Input: part model. Units: mm. Frame: model coordinates. A direction names the side the tool comes from. Coordinates: 2 decimals unless noted, no trailing zeros. Write each loop counter-clockwise with the first axis right and the second up, starting at its lowest first coordinate (ties: lowest second). Pieces come first, ordered by that corner, then holes. Notation, with made-up numbers: (84, 26) - (133, 26) arc R31 ccw to (133, 64) - close; hole circle Ø2 at (74.5, -17.5). An arc over 180 degrees is marked (long way). Use CSV: the item, a comma, the result in double quotes.
```python
from build123d import *

# Parameters (mm, degrees)
CROQUIS1_R              = 2
SALIENTE_EXTRUIR1_DEPTH = 7
SALIENTE_EXTRUIR2_DEPTH = 5
SALIENTE_EXTRUIR3_DEPTH = 5
SALIENTE_EXTRUIR4_DEPTH = 5
CROQUIS6_R              = 2
CORTAR_EXTRUIR1_DEPTH   = 20
SALIENTE_EXTRUIR5_DEPTH = 5
CROQUIS8_R              = 2
CORTAR_EXTRUIR3_DEPTH   = 20
CORTAR_EXTRUIR4_DEPTH   = 20
CROQUIS10_R             = 2
CORTAR_EXTRUIR5_DEPTH   = 5
CROQUIS12_R             = 2
CORTAR_EXTRUIR6_DEPTH   = 5
CROQUIS13_R             = 2
CORTAR_EXTRUIR7_DEPTH   = 45


with BuildPart() as part:
    # Croquis1 → Saliente-Extruir1 (new body)
    with BuildSketch(Plane.XY):
        with BuildLine():
            Line((0, 161.361306161), (59.639031754, 161.361306161))
            ThreePointArc((59.639031754, 161.361306161), (66.710099565, 158.432373972), (69.639031754, 151.361306161))
            Line((69.639031754, 151.361306161), (69.639031754, 150.370999495))
            ThreePointArc((69.639031754, 150.370999495), (70.657777859, 141.400946832), (73.662123993, 132.887804479))
            ThreePointArc((73.662123993, 132.887804479), (90.138531177, 101.602103147), (108.605347016, 71.44843315))
            ThreePointArc((108.605347016, 71.44843315), (129.868212527, 5.85212568), (114.591350051, -61.390736219))
            ThreePointArc((114.591350051, -61.390736219), (94.163470567, -82.020942746), (65.787006352, -88.15934321))
            ThreePointArc((65.787006352, -88.15934321), (108.340691896, -19.034034767), (91.89683209, 60.456366511))
            ThreePointArc((91.89683209, 60.456366511), (70.390740309, 96.854398001), (52.489257919, 135.15407957))
            ThreePointArc((52.489257919, 135.15407957), (48.807435802, 139.665754791), (43.236427549, 141.361306161))
            Line((43.236427549, 141.361306161), (0, 141.361306161))
            Line((0, 141.361306161), (0, 161.361306161))
        make_face()
        with Locations((59.639031754, 151.361306161)):
            Circle(CROQUIS1_R, mode=Mode.SUBTRACT)
    extrude(amount=SALIENTE_EXTRUIR1_DEPTH)

    # Croquis2 → Saliente-Extruir2 (add)
    with BuildSketch(Plane.XY.offset(7)):
        with BuildLine():
            Line((54.416767437, 141.361306161), (43.236427549, 141.361306161))
            ThreePointArc((43.236427549, 141.361306161), (48.807435802, 139.665754791), (52.489257919, 135.15407957))
            ThreePointArc((52.489257919, 135.15407957), (70.390740309, 96.854398001), (91.89683209, 60.456366511))
            ThreePointArc((91.89683209, 60.456366511), (108.340691896, -19.034034767), (65.787006352, -88.15934321))
            ThreePointArc((65.787006352, -88.15934321), (69.834622147, -88.304656697), (73.881004217, -88.128299745))
            ThreePointArc((73.881004217, -88.128299745), (113.782985393, -16.686288834), (96.073960822, 63.204383171))
            ThreePointArc((96.073960822, 63.204383171), (74.813060375, 99.187440057), (57.115673105, 137.050466275))
            ThreePointArc((57.115673105, 137.050466275), (55.950260204, 139.321108873), (54.416767437, 141.361306161))
        make_face()
    extrude(amount=SALIENTE_EXTRUIR2_DEPTH)

    # Croquis4 → Saliente-Extruir4 (add)
    with BuildSketch(Plane.XY.offset(7)):
        with BuildLine():
            Line((69.639031754, 151.361306161), (69.639031754, 150.370999495))
            ThreePointArc((69.639031754, 150.370999495), (69.896834815, 145.836930406), (70.666920879, 141.361306161))
            Line((70.666920879, 141.361306161), (54.416767437, 141.361306161))
            Line((54.416767437, 141.361306161), (0, 141.361306161))
            Line((0, 141.361306161), (0, 161.361306161))
            Line((0, 161.361306161), (59.639031754, 161.361306161))
            ThreePointArc((59.639031754, 161.361306161), (66.710099565, 158.432373972), (69.639031754, 151.361306161))
        make_face()
    extrude(amount=SALIENTE_EXTRUIR4_DEPTH)

    # Croquis6 → Cortar-Extruir1 (cut)
    with BuildSketch(Plane(origin=(0, 0, 0), x_dir=(-1, 0, 0), z_dir=(0, 0, -1))):
        with Locations((-59.639031754, 151.361306161)):
            Circle(CROQUIS6_R)
    extrude(amount=-CORTAR_EXTRUIR1_DEPTH, mode=Mode.SUBTRACT)



with BuildPart() as body_2:
    # Croquis3 → Saliente-Extruir3 (new body)
    with BuildSketch(Plane(origin=(0, 0, 0), x_dir=(-1, 0, 0), z_dir=(0, 0, -1))):
        with BuildLine():
            Line((-43.236427549, 141.361306161), (-54.416767437, 141.361306161))
            ThreePointArc((-54.416767437, 141.361306161), (-55.950260204, 139.321108873), (-57.115673105, 137.050466275))
            ThreePointArc((-57.115673105, 137.050466275), (-74.813060375, 99.187440057), (-96.073960822, 63.204383171))
            ThreePointArc((-96.073960822, 63.204383171), (-113.782985393, -16.686288834), (-73.881004217, -88.128299745))
            ThreePointArc((-73.881004217, -88.128299745), (-69.834622147, -88.304656697), (-65.787006352, -88.15934321))
            ThreePointArc((-65.787006352, -88.15934321), (-108.340691896, -19.034034767), (-91.89683209, 60.456366511))
            ThreePointArc((-91.89683209, 60.456366511), (-70.390740309, 96.854398001), (-52.489257919, 135.15407957))
            ThreePointArc((-52.489257919, 135.15407957), (-48.807435802, 139.665754791), (-43.236427549, 141.361306161))
        make_face()
    extrude(amount=SALIENTE_EXTRUIR3_DEPTH)


with BuildPart() as part_1:
    add(part.part)

    add(body_2.part)  # Saliente-Extruir5 merges body 2
    # Croquis7 → Saliente-Extruir5 (add)
    with BuildSketch(Plane(origin=(0, 0, 0), x_dir=(-1, 0, 0), z_dir=(0, 0, -1))):
        with BuildLine():
            Line((0, 161.361306161), (-59.639031754, 161.361306161))
            ThreePointArc((-59.639031754, 161.361306161), (-66.710099565, 158.432373972), (-69.639031754, 151.361306161))
            Line((-69.639031754, 151.361306161), (-69.639031754, 150.370999495))
            ThreePointArc((-69.639031754, 150.370999495), (-69.896834815, 145.836930406), (-70.666920879, 141.361306161))
            Line((-70.666920879, 141.361306161), (-54.416767437, 141.361306161))
            Line((-54.416767437, 141.361306161), (0, 141.361306161))
            Line((0, 141.361306161), (0, 161.361306161))
        make_face()
    extrude(amount=SALIENTE_EXTRUIR5_DEPTH)

    # Croquis8 → Cortar-Extruir3 (cut)
    with BuildSketch(Plane.XY.offset(12)):
        with Locations((59.639031754, 151.361306161)):
            Circle(CROQUIS8_R)
    extrude(amount=-CORTAR_EXTRUIR3_DEPTH, mode=Mode.SUBTRACT)

    # Croquis9 → Cortar-Extruir4 (cut)
    with BuildSketch(Plane.XY.offset(12)):
        with BuildLine():
            ThreePointArc((26.006407842, 141.361306161), (16.006407842, 151.361306161), (26.006407842, 161.361306161))
            Line((26.006407842, 161.361306161), (0, 161.361306161))
            Line((0, 161.361306161), (0, 141.361306161))
            Line((0, 141.361306161), (26.006407842, 141.361306161))
        make_face()
    extrude(amount=-CORTAR_EXTRUIR4_DEPTH, mode=Mode.SUBTRACT)

    # Croquis10 → Cortar-Extruir5 (cut)
    with BuildSketch(Plane.XY.offset(12)):
        with BuildLine():
            Line((41.006407842, 161.361306161), (26.006407842, 161.361306161))
            ThreePointArc((26.006407842, 161.361306161), (16.006407842, 151.361306161), (26.006407842, 141.361306161))
            Line((26.006407842, 141.361306161), (41.006407842, 141.361306161))
            Line((41.006407842, 141.361306161), (41.006407842, 161.361306161))
        make_face()
        with Locations((26.006407842, 151.361306161)):
            Circle(CROQUIS10_R, mode=Mode.SUBTRACT)
    extrude(amount=-CORTAR_EXTRUIR5_DEPTH, mode=Mode.SUBTRACT)

    # Croquis12 → Cortar-Extruir6 (cut)
    with BuildSketch(Plane(origin=(0, 0, -5), x_dir=(-1, 0, 0), z_dir=(0, 0, -1))):
        with BuildLine():
            Line((-26.006407842, 161.361306161), (-41.006407842, 161.361306161))
            Line((-41.006407842, 161.361306161), (-41.006407842, 141.361306161))
            Line((-41.006407842, 141.361306161), (-26.006407842, 141.361306161))
            ThreePointArc((-26.006407842, 141.361306161), (-16.006407842, 151.361306161), (-26.006407842, 161.361306161))
        make_face()
        with Locations((-26.006407842, 151.361306161)):
            Circle(CROQUIS12_R, mode=Mode.SUBTRACT)
    extrude(amount=-CORTAR_EXTRUIR6_DEPTH, mode=Mode.SUBTRACT)

    # Croquis13 → Cortar-Extruir7 (cut)
    with BuildSketch(Plane(origin=(0, 0, -5), x_dir=(-1, 0, 0), z_dir=(0, 0, -1))):
        with Locations((-26.006407842, 151.361306161)):
            Circle(CROQUIS13_R)
    extrude(amount=-CORTAR_EXTRUIR7_DEPTH, mode=Mode.SUBTRACT)


solid = part_1.part
```
(1) Ray query, probe 1 along Y at (x, z) = (58, -1); probe 2 along Z at (x, y) = (39, 144); probe 3 along Y at (x, z) = (60, 6.5). Return the intervals inside material, ascending. Write a range as from..to.
Check values:
probe 1,"122.3..134.91, 141.36..150.22, 152.51..161.36"
probe 2,"0..7"
probe 3,"117.9..149.39, 153.33..161.35"
(2) Cut plane B-B on x = 82.5. Return loops of the section in (y, z), and give its area (3 significant figures).
Check values:
outline,"(-86.66, 0) - (-80.12, 0) - (-80.12, -5) - (-72.76, -5) - (-72.76, 12) - (-80.12, 12) - (-80.12, 7) - (-86.66, 7) - close; (75.39, -5) - (85.24, -5) - (85.24, 0) - (115.5, 0) - (115.5, 7) - (85.24, 7) - (85.24, 12) - (75.39, 12) - close"
area,"550 mm^2"
(3) Reachability of faces 1 (the flat face through (37, 141.361, 4)), 2 (the cylindrical face through (70.67, 96.33, 3.62)), 3 (the flat face through (112, 27, 0)), 4 (the flat face through (112, 27, 7)), 5 (the flat face through (41.006, 151, 10)) from +Z, -Z, +X, -X, +Y, -Y: full face, straight path, thin tool, end or side. Return the list, or none.
Check values:
face 1,"+Z, -Z, -X, -Y"
face 2,"+Z, -Z, -X"
face 3,"-Z, +X"
face 4,"+Z, +X"
face 5,"+Z, -X, +Y, -Y"
(4) Cut plane C-C on y = 84.5. Return loops of the section in (x, z).
Check values:
outline,"(77.16, -5) - (82.93, -5) - (82.93, 0) - (100.28, 0) - (100.28, 7) - (82.93, 7) - (82.93, 12) - (77.16, 12) - close"
(5) Cut plane D-D on x = 101. Return loops of the section in (y, z).
Check values:
outline,"(-77.52, 0) - (-54.99, 0) - (-54.99, -5) - (-43.58, -5) - (-43.58, 12) - (-54.99, 12) - (-54.99, 7) - (-77.52, 7) - close; (43.58, -5) - (54.99, -5) - (54.99, 0) - (83.34, 0) - (83.34, 7) - (54.99, 7) - (54.99, 12) - (43.58, 12) - close"
(6) Cut plane A-A on z = 9.25. Return loops of the section in (x, y), and give its area (3 significant figures).
Check values:
outline,"(41.01, 141.36) - (43.24, 141.36) arc R10 cw to (52.49, 135.15) arc R438.56 ccw to (91.9, 60.46) arc R110 cw to (65.79, -88.16) arc R51 ccw to (73.88, -88.13) arc R115 ccw to (96.07, 63.2) arc R433.56 cw to (57.12, 137.05) arc R15 ccw to (54.42, 141.36) - (70.67, 141.36) arc R40 cw to (69.64, 150.37) - (69.64, 151.36) arc R10 ccw to (59.64, 161.36) - (41.01, 161.36) - close; hole circle Ø4 at (59.64, 151.36)"
area,"1,830 mm^2"
(7) Draft query along Y for faces 6 (the cylindrical face through (113.947, -15.527, -2.465)), 7 (the flat face through (63, 141.361, 9)), 8 (the cylindrical face through (55.97, 139.29, 9.46)), 9 (the flat face through (28.3, 151.5, 7)). Return one class per face: pulls with the +Y half, pulls with the -Y half, needs draft (parallel to the pull), parting line crosses it, or undercut.
Check values:
face 6,"parting line crosses it"
face 7,"undercut"
face 8,"undercut"
face 9,"needs draft"
(8) Pin query (flat end, axial travel): pin 1 Ø2.5 at (y, z) = (149.5, -3) entering from -X; pin 2 Ø6 at (x, z) = (100, 8.5) entering from +Y; pin 3 Ø3.5 at (x, y) = (26.01, 151.36) entering from +Z; pin 4 Ø2 at (x, z) = (49.5, 10) entering from -Y. Return the tip coordinate at first contact, or that it passes through.
Check values:
pin 1,"x = 41.01"
pin 2,"y = 89.21"
pin 3,"through"
pin 4,"y = 138.23"
